Source: CAD feature listing. Evaluate the final solid. Frame: model axes, mm. A direction names the side the tool comes from. Give positions to 0.01 mm unless a question says otherwise; leave off trailing zeros. Write each loop counter-clockwise with the first axis right and the second up, starting at its lowest first coordinate (ties: lowest second). Pieces come first, ordered by that corner, then holes. Notation, with made-up numbers: M 42.5,-9 L 68.5,-9 A31 cw 68.5,24 Z; hole C -23,28.5 d10. An arc over 180 degrees is marked long. Return JSON: item names as keys, results as strings.
```python
from build123d import *

# Parameters (mm, degrees)
F0_W     = 45
F0_H     = 22
F0_W_2   = 40
F0_H_2   = 18
F1_DEPTH = 10
F2_DEPTH = 24
F3_R     = 2
F4_DEPTH = 10


with BuildPart() as f1:
    # F0 (on Top) → F1 (new body)
    with BuildSketch(Plane.XY):
        with Locations((-36.311314, -9.456807)):
            Rectangle(F0_W, F0_H)
        with Locations((-36.311314, -9.456807)):
            Rectangle(F0_W_2, F0_H_2, mode=Mode.SUBTRACT)
        with Locations((-36.311314, -9.456807)):
            Rectangle(F0_W_2, F0_H_2)
    extrude(amount=F1_DEPTH)

    # F0 (on Top) → F2 (join)
    with BuildSketch(Plane.XY):
        with Locations((-36.311314, -9.456807)):
            Rectangle(F0_W_2, F0_H_2)
    extrude(amount=-F2_DEPTH)

    # F3 (on face) → F4 (join)
    with BuildSketch(Plane(origin=(0, 0, -24), x_dir=(1, 0, 0), z_dir=(0, 0, -1))):
        with Locations((-46.311314, 16.456807)):
            Circle(F3_R)
        with Locations((-46.311314, 11.806807)):
            Circle(F3_R)
        with Locations((-46.311314, 7.156807)):
            Circle(F3_R)
        with Locations((-46.311314, 2.506807)):
            Circle(F3_R)
        with Locations((-26.311314, 16.456807)):
            Circle(F3_R)
        with Locations((-26.311314, 11.806807)):
            Circle(F3_R)
        with Locations((-26.311314, 7.156807)):
            Circle(F3_R)
        with Locations((-26.311314, 2.506807)):
            Circle(F3_R)
    extrude(amount=F4_DEPTH)


solid = f1.part
```
1) Cut plane B-B, the plane x = -29.5. Return the cut outline in (y, z), then the cut area to 3 significant figures.
Numbers:
{"outline": "M -20.46,0 L -18.46,0 L -18.46,-24 L -0.46,-24 L -0.46,0 L 1.54,0 L 1.54,10 L -20.46,10 Z", "area": "652 mm²"}
2) Cut plane D-D, the plane y = -6. Return the cut outline in (x, z).
Numbers:
{"outline": "M -58.81,0 L -56.31,0 L -56.31,-24 L -47.94,-24 L -47.94,-34 L -44.68,-34 L -44.68,-24 L -27.94,-24 L -27.94,-34 L -24.68,-34 L -24.68,-24 L -16.31,-24 L -16.31,0 L -13.81,0 L -13.81,10 L -58.81,10 Z"}
3) Cut plane A-A, the plane z = -25.5. Return the cut outline in (x, y), then the cut area to 3 significant figures.
Numbers:
{"outline": "C -46.31,-16.46 d4; C -46.31,-11.81 d4; C -46.31,-7.16 d4; C -46.31,-2.51 d4; C -26.31,-16.46 d4; C -26.31,-11.81 d4; C -26.31,-7.16 d4; C -26.31,-2.51 d4", "area": "101 mm²"}
4) Draft query along Y for faces 6 (the face through (-37, -0.457, -12)), 7 (the face through (-13.811, -10, 5)), 8 (the face through (-48.31, -2.59, -28.93)). Return one class per face: released by +Y, released by -Y, zero draft, split by the parting line, or undercut.
Numbers:
{"face 6": "released by +Y", "face 7": "zero draft", "face 8": "undercut"}
5) Contact query for flat-ended pins moving along their axis: pin 1 Ø6 at (y, z) = (-7, -8.5) entering from -X; pin 2 Ø4 at (x, z) = (-31.5, -5.5) entering from -Y; pin 3 Ø19 at (x, z) = (-44.5, -10) entering from +Y; pin 4 Ø12 at (x, z) = (-22, -3.5) entering from +Y. Output: stop coordinate, or through.
Numbers:
{"pin 1": "stops at x = -56.31", "pin 2": "stops at y = -18.46", "pin 3": "stops at y = -0.46", "pin 4": "stops at y = 1.54"}
6) Cut plane C-C, the plane y = -12.75. Return the cut outline in (x, z), then the cut area to 3 significant figures.
Numbers:
{"outline": "M -58.81,0 L -56.31,0 L -56.31,-24 L -48.07,-24 L -48.07,-34 L -44.55,-34 L -44.55,-24 L -28.07,-24 L -28.07,-34 L -24.55,-34 L -24.55,-24 L -16.31,-24 L -16.31,0 L -13.81,0 L -13.81,10 L -58.81,10 Z", "area": "1,480 mm²"}
7) Line query: line 1 (Y direction, x = -25, z = -30); line 2 (Z direction, x = -43.5, y = -12.5); line 3 (Y direction, x = -48.5, z = -5). Output: solid intervals per line, ascending. Write a range as [from, to].
Numbers:
{"line 1": "y = [-17.97, -14.95], [-13.32, -10.3], [-8.67, -5.65], [-4.02, -1]", "line 2": "z = [-24, 10]", "line 3": "y = [-18.46, -0.46]"}
8) Set-up query: faces 1 (the face through (-48.31, -16.54, -28.93)), 2 (the face through (-26, -3, -34)), 3 (the face through (-16.311, -10, -12)), 4 (the face through (-58.811, -10, 5)), 5 (the face through (-56.311, -10, -12)). Return all of +Z, -Z, +X, -X, +Y, -Y with unobstructed straight access to the full face (end or side cutting, diameter ignored); none if empty.
Numbers:
{"face 1": "-Z", "face 2": "-Z, +X, -X, +Y, -Y", "face 3": "-Z, +X, +Y, -Y", "face 4": "+Z, -Z, -X, +Y, -Y", "face 5": "-Z, -X, +Y, -Y"}
